For this review, take the finished solid that the model builds, in its own axes (mm). Face numbers are marked on the shaded views. A direction names the side the tool comes from. Give positions to 0.01 mm unless a question says otherwise; leave off trailing zeros. Write each loop counter-clockwise with the first axis right and the second up, starting at its lowest first coordinate (ties: lowest second). Pieces come first, ordered by that corner, then holes. Notation, with made-up numbers: M 50.5,68.25 L 68.5,68.25 A13 ccw 68.5,86.25 Z; hole C 12.25,7 d4. An arc over 180 degrees is marked long. Write item = value, one per line.
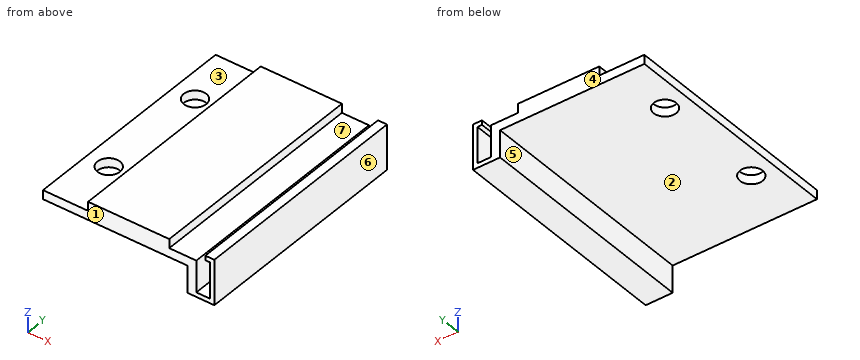
```python
from build123d import *

# Parameters (mm, degrees)
ESQUISSE1_W             = 10
ESQUISSE1_H             = 50
ESQUISSE1_R             = 2.5
ESQUISSE1_W_2           = 2
BOSS_EXTRU_1_DEPTH      = 2
ESQUISSE2_W             = 2
ESQUISSE2_H             = 50
BOSS_EXTRU_2_DEPTH      = 2
ESQUISSE3_W             = 4
ESQUISSE3_H             = 50
BOSS_EXTRU_3_DEPTH      = 22
ESQUISSE4_W             = 2
ESQUISSE4_H             = 50
BOSS_EXTRU_4_DEPTH      = 6
ESQUISSE5_W             = 2
ESQUISSE5_H             = 50
ENL_V_MAT_EXTRU_1_DEPTH = 6
ESQUISSE6_W             = 1
ESQUISSE6_H             = 50
BOSS_EXTRU_5_DEPTH      = 4
ESQUISSE7_W             = 1
ESQUISSE7_H             = 50
BOSS_EXTRU_6_DEPTH      = 9
ESQUISSE8_W             = 1
ESQUISSE8_H             = 50
BOSS_EXTRU_7_DEPTH      = 1


with BuildPart() as part:
    # Esquisse1 → Boss.-Extru.1 (new body)
    with BuildSketch(Plane.XY):
        with Locations((5, 25)):
            Rectangle(ESQUISSE1_W, ESQUISSE1_H)
        with Locations((5, 12.5)):
            Circle(ESQUISSE1_R, mode=Mode.SUBTRACT)
        with Locations((5, 37.5)):
            Circle(ESQUISSE1_R, mode=Mode.SUBTRACT)
        with Locations((11, 25)):
            Rectangle(ESQUISSE1_W_2, ESQUISSE1_H)
    extrude(amount=BOSS_EXTRU_1_DEPTH)

    # Esquisse2 → Boss.-Extru.2 (add)
    with BuildSketch(Plane.XY.offset(2)):
        with Locations((11, 25)):
            Rectangle(ESQUISSE2_W, ESQUISSE2_H)
    extrude(amount=BOSS_EXTRU_2_DEPTH)

    # Esquisse3 → Boss.-Extru.3 (add)
    with BuildSketch(Plane(origin=(12, 0, 0), x_dir=(0, 0, -1), z_dir=(1, 0, 0))):
        with Locations((-2, 25)):
            Rectangle(ESQUISSE3_W, ESQUISSE3_H)
    extrude(amount=BOSS_EXTRU_3_DEPTH)

    # Esquisse4 → Boss.-Extru.4 (add)
    with BuildSketch(Plane(origin=(0, 0, 0), x_dir=(-1, 0, 0), z_dir=(0, 0, -1))):
        with Locations((-33, 25)):
            Rectangle(ESQUISSE4_W, ESQUISSE4_H)
    extrude(amount=BOSS_EXTRU_4_DEPTH)

    # Esquisse5 → Enlèv. mat.-Extru.1 (cut)
    with BuildSketch(Plane(origin=(34, 0, 0), x_dir=(0, 0, -1), z_dir=(1, 0, 0))):
        with Locations((-3, 25)):
            Rectangle(ESQUISSE5_W, ESQUISSE5_H)
    extrude(amount=-ENL_V_MAT_EXTRU_1_DEPTH, mode=Mode.SUBTRACT)

    # Esquisse6 → Boss.-Extru.5 (add)
    with BuildSketch(Plane(origin=(34, 0, 0), x_dir=(0, 0, -1), z_dir=(1, 0, 0))):
        with Locations((5.5, 25)):
            Rectangle(ESQUISSE6_W, ESQUISSE6_H)
    extrude(amount=BOSS_EXTRU_5_DEPTH)

    # Esquisse7 → Boss.-Extru.6 (add)
    with BuildSketch(Plane.XY.offset(-5)):
        with Locations((37.5, 25)):
            Rectangle(ESQUISSE7_W, ESQUISSE7_H)
    extrude(amount=BOSS_EXTRU_6_DEPTH)

    # Esquisse8 → Boss.-Extru.7 (add)
    with BuildSketch(Plane.ZY.offset(-37)):
        with Locations((3.5, 25)):
            Rectangle(ESQUISSE8_W, ESQUISSE8_H)
    extrude(amount=BOSS_EXTRU_7_DEPTH)


solid = part.part
```
1. Insertion check: P1, Ø8, axis at x = 5, y = 37.5, coming from the -Z side; P2, Ø3, axis at y = 8, z = -2.5, coming from the -X side; P3, Ø1.5, axis at x = 35, y = 29.5, coming from the +Z side; P4, Ø5, axis at x = 28.5, z = -0.5, coming from the +Y side. Each pin has a flat end and moves straight along its axis. Give the tip position at first contact, or say it passes through.
Responses:
P1 = 0
P2 = 32
P3 = -5
P4 = 50
2. We need section B-B, the plane z = -2.5. Write out the cut boundary in (x, y).
Responses:
outline = M 32,0 L 34,0 L 34,50 L 32,50 Z; M 37,0 L 38,0 L 38,50 L 37,50 Z
3. We need section D-D, the plane y = 29.5. Write out the cut boundary in (x, z), then the cut area to 3 significant figures.
Responses:
outline = M 0,0 L 32,0 L 32,-6 L 38,-6 L 38,4 L 36,4 L 36,3 L 37,3 L 37,-5 L 34,-5 L 34,2 L 28,2 L 28,4 L 10,4 L 10,2 L 0,2 Z
area = 130 mm2
4. Machinability: for the marked faces 1, 2 and 3, which of the approach directions +Z, -Z, +X, -X, +Y, -Y give a long, thin tool a straight path to every point of the face, cutting with its end or side? Answer none if there is none.
Responses:
face_1 = +Z, -Z, +X, -X, -Y
face_2 = -Z, -X, +Y, -Y
face_3 = +Z, -X, +Y, -Y
5. We need section A-A, the plane x = 5. Write out the cut boundary in (y, z).
Responses:
outline = M 0,0 L 10,0 L 10,2 L 0,2 Z; M 15,0 L 35,0 L 35,2 L 15,2 Z; M 40,0 L 50,0 L 50,2 L 40,2 Z
6. For line 1 along X through (y, z) = (17, 0.25); line 2 along X through (y, z) = (31.5, -4.75); line 3 along Y through (x, z) = (5, 1), list the stretches that pass through material, from the lowest coordinate up. Write a range as from..to.
Responses:
line_1 = 0..34, 37..38
line_2 = 32..34, 37..38
line_3 = 0..10, 15..35, 40..50
7. The part is to be moulded in two halves that separate along X. For the marked faces 4, 5, 6 and 7, say which applies: +X half, -X half, draft (parallel to the pull), parting line (faces both ways), or undercut.
Responses:
face_4 = draft
face_5 = -X half
face_6 = +X half
face_7 = undercut
8. We need section C-C, the plane y = 12.5. Write out the cut boundary in (x, z).
Responses:
outline = M 0,0 L 2.5,0 L 2.5,2 L 0,2 Z; M 7.5,0 L 32,0 L 32,-6 L 38,-6 L 38,4 L 36,4 L 36,3 L 37,3 L 37,-5 L 34,-5 L 34,2 L 28,2 L 28,4 L 10,4 L 10,2 L 7.5,2 Z
